Could you check a few things on this drawing? It's one solid part, dimensions in mm from its lowest x, y, z. A direction names the side the tool comes from. Give positions to 0.01 mm unless a question says otherwise; leave off trailing zeros. Write each loop counter-clockwise with the first axis right and the second up, starting at its lowest first coordinate (ties: lowest second). Pieces come first, ordered by that corner, then holes.
1. Suppose I cut it at C-C (z = 18.75). Please give me the cut outline in (x, y).
2. On a 3-axis mill with a long thin cutter (end or side, diameter ignored), from which of +Z, -Z, +X, -X, +Y, -Y can I reach the whole of each face in a straight line? I mean the marked faces 1, 2, 3, 4 and 5. Say none if no direction works.
3. Suppose I cut it at A-A (y = 12.7). Please give me the cut outline in (x, z) (3 decimals).
4. Suppose I cut it at D-D (z = 14.5). Please give me the cut outline in (x, y) (3 decimals), and give its area (3 significant figures).
5. If I drill on probe 1 along Z at (x, y) = (11.5, 4); probe 2 along X at (y, z) = (12.75, 10.25); probe 3 along X at (y, z) = (12.25, 14.75), over which ranges is the centre line in solid material (lowest first)?
6. Suppose I cut it at B-B (x = 28). Please give me the cut outline in (y, z) (3 decimals).
7. I'm going to push flat-ended pins straight in: pin 1 (2 mm diameter, centred on x = 8.5, y = 12.5, fed in from -Z); pin 2 (1.5 mm diameter, centred on x = 7.5, z = 14, fed in from +Y); pin 3 (7.5 mm diameter, centred on x = 6.5, y = 18.5, fed in from +Z); pin 4 (8 mm diameter, centred on x = 9.5, y = 7.5, fed in from -Z). Where does each tip first touch, or does it pass through?
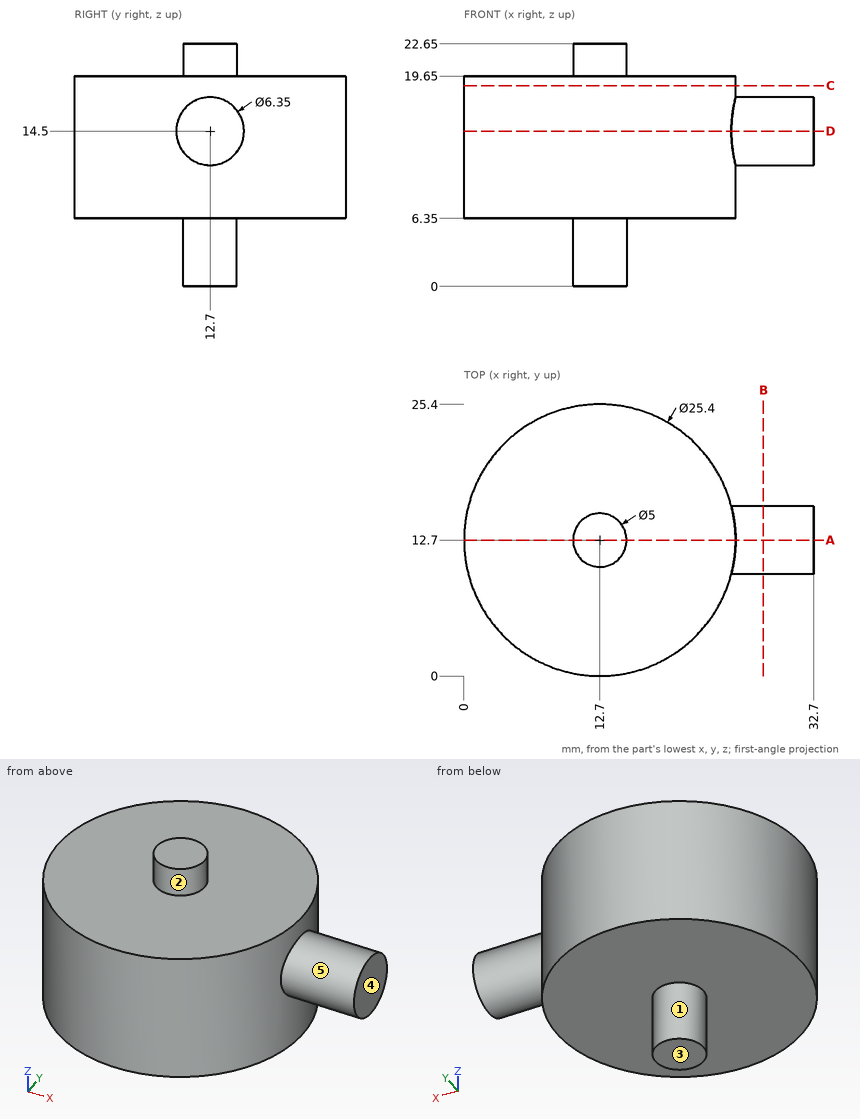
Checks:
1. outline: circle Ø25.4 at (12.7, 12.7)
2. face 1: -Z
2. face 2: +Z
2. face 3: -Z, +X, -X, +Y, -Y
2. face 4: +Z, -Z, +X, +Y, -Y
2. face 5: +X
3. outline: (0, 6.35) - (10.2, 6.35) - (10.2, 0) - (15.2, 0) - (15.2, 6.35) - (25.4, 6.35) - (25.4, 11.325) - (32.7, 11.325) - (32.7, 17.675) - (25.4, 17.675) - (25.4, 19.65) - (15.2, 19.65) - (15.2, 22.65) - (10.2, 22.65) - (10.2, 19.65) - (0, 19.65) - close
4. outline: (24.997, 9.525) - (32.7, 9.525) - (32.7, 15.875) - (24.997, 15.875) arc R12.7 ccw (long way) to start
4. area: 554 mm2
5. probe 1: z = 6.35 to 19.65
5. probe 2: x = 0 to 25.4
5. probe 3: x = 0.01 to 32.7
6. outline: circle Ø6.35 at (12.7, 14.5)
7. pin 1: stops at z = 6.35
7. pin 2: stops at y = 24.59
7. pin 3: stops at z = 19.65
7. pin 4: stops at z = 0
